Build history of the part. All positions in model axes, mm. A direction names the side the tool comes from. Coordinates: 2 decimals unless noted, no trailing zeros. Write each loop counter-clockwise with the first axis right and the second up, starting at its lowest first coordinate (ties: lowest second). Pieces come first, ordered by that corner, then holes.
```python
from build123d import *

# Parameters (mm, degrees)
SKETCH_1_R          = 3
EXTRUDE_1_DEPTH     = 0.8
CUT_EXTRUDE_1_DEPTH = 0.5


# Read off the part's stored shape, not the designer's step: M3 机械螺纹 螺柱3
with BuildPart() as part:
    # 草图1 → 凸台-拉伸1 (new body)
    with BuildSketch(Plane(origin=(0, 0, 0), x_dir=(1, 0, 0), z_dir=(0, 1, 0))):
        with Locations(Location((0, 0, 0), (0, 0, 270))):
            Circle(SKETCH_1_R)
    extrude(amount=EXTRUDE_1_DEPTH)

    # M3 机械螺纹 螺柱3 outline → M3 机械螺纹 螺柱3 (revolve)
    with BuildSketch(Plane.XY):
        Polygon((1.2295, 8.8), (0, 8.8), (0, 0.8), (1.5, 0.8), (1.5, 8.5295), align=None)
    revolve(axis=Axis((0, 0, 0), (0, 1, 0)))

    # 草图8 → 切除-拉伸1 (cut)
    with BuildSketch(Plane.XZ):
        Polygon((1.154700538, 0), (0.577350269, 1), (-0.577350269, 1), (-1.154700538, 0), (-0.577350269, -1), (0.577350269, -1), align=None)
    extrude(amount=-CUT_EXTRUDE_1_DEPTH, mode=Mode.SUBTRACT)


solid = part.part
```
1. Saw through at D-D on z = 2.3. List the corners of the cut face in (x, y).
Computed values:
outline: (-1.93, 0) - (1.93, 0) - (1.93, 0.8) - (-1.93, 0.8) - close
2. Saw through at C-C on y = 2.25. List the corners of the cut face in (x, z), plus the area to 3 significant figures.
Computed values:
outline: circle Ø3 at (0, 0)
area: 7.07 mm2
3. Flat gauge pins, fed straight in: pin 1 (1.5 mm diameter, centred on y = 7, z = -1, fed in from +X); pin 2 (1.6 mm diameter, centred on x = 0, z = 0.5, fed in from -Y); pin 3 (2 mm diameter, centred on x = 2.5, y = 1, fed in from +Z); pin 4 (1 mm diameter, centred on y = 5.5, z = 0, fed in from -X). Where does each tip first touch, or does it go through?
Computed values:
pin 1: stops at x = 1.48
pin 2: stops at y = 0
pin 3: stops at z = 2.59
pin 4: stops at x = -1.5
4. Saw through at B-B on z = -2.4. List the corners of the cut face in (x, y).
Computed values:
outline: (-1.8, 0) - (1.8, 0) - (1.8, 0.8) - (-1.8, 0.8) - close
5. 3-axis set-ups, long thin cutter, end or side, ignore diameter. For faces 1 (the face through (-1.5, 4.72, -0.07)), 2 (the face through (0, 0, 1.3)): which of +Z, -Z, +X, -X, +Y, -Y reach the whole face in a straight line?
Computed values:
face 1: +Y
face 2: +Z, -Z, +X, -X, -Y
6. Mould opens along Z. For faces 3 (the face through (-1.3, 0.8, 1.3)), 4 (the face through (0, 0.5, 0)), 5 (the face through (0.9, 0.39, 2.86)) say: +Z half, -Z half, draft (parallel to the pull), parting line (faces both ways), or undercut.
Computed values:
face 3: draft
face 4: undercut
face 5: parting line
7. Saw through at A-A on x = 0. List the corners of the cut face in (y, z), plus the area to 3 significant figures.
Computed values:
outline: (0, -3) - (0.8, -3) - (0.8, -1.5) - (8.53, -1.5) - (8.8, -1.23) - (8.8, 1.23) - (8.53, 1.5) - (0.8, 1.5) - (0.8, 3) - (0, 3) - (0, 1) - (0.5, 1) - (0.5, -1) - (0, -1) - close
area: 27.7 mm2
8. Probe line 1 along Y through (x, z) = (1.25, 1.65); line 2 along Y through (x, z) = (0.7, 0.7); line 3 along Z through (x, y) = (0.05, 6.5). List the from-to ranges inside material, lowest first.
Computed values:
line 1: y = 0 to 0.8
line 2: y = 0.5 to 8.8
line 3: z = -1.5 to 1.5
